Read the model definition and answer for the solid it produces. Units are mm, in the model's axes. Face numbers are marked on the shaded views. Round coordinates to 2 decimals unless told otherwise and drop trailing zeros. Loops run counter-clockwise (first coordinate to the right, second up) from the corner with the lowest first, then second, coordinate; pieces in that order, holes last. Notation, with made-up numbers: M -38,69 L 11,69 A11 ccw 11,87 Z; hole C 2.5,58.5 d4. An arc over 180 degrees is marked long. Write each question's results on one line, items separated by ' | '.
```python
from build123d import *

# Parameters (mm, degrees)
SKETCH1_R                  = 8.89
BOSS_EXTRUDE1_DEPTH        = 38.1
F_3_0MM_DOWEL_HOLE2_D      = 3.5
F_12_CLEARANCE_HOLE1_D     = 5.7912
F_12_CLEARANCE_HOLE1_DEPTH = 19.05
F_12_CLEARANCE_HOLE1_TIP   = 1.739852008


# Read off the part's stored shape, not the designer's step: CBORE for #2 Button Head Cap Screw1
with BuildPart() as part:
    # Sketch1 → Boss-Extrude1 (new body)
    with BuildSketch(Plane(origin=(0, 0, 0), x_dir=(1, 0, 0), z_dir=(0, 1, 0))):
        with Locations(Location((0, 0, 0), (0, 0, 90))):
            Circle(SKETCH1_R)
    extrude(amount=BOSS_EXTRUDE1_DEPTH)

    # Ø3.0mm Dowel Hole2 (through all)
    with Locations(Plane(origin=(0, 38.1, 0), x_dir=(1, 0, 0), z_dir=(0, 1, 0))):
        with Locations((0, 0)):
            Hole(F_3_0MM_DOWEL_HOLE2_D / 2)

    # CBORE for #2 Button Head Cap Screw1 outl → CBORE for #2 Button Head Cap Screw1 (revolve, cut)
    with BuildSketch(Plane(origin=(0, 5.08, 0), x_dir=(0, 1, 0), z_dir=(0, 0, -1))):
        Polygon((1.35255, 6.9596), (2.70637, 6.9596), (2.70637, 8.890055176), (0, 8.890055176), (0, 1.110061146), (1.35255, 1.110061146), align=None)
    revolve(axis=Axis((0, 5.08, 0), (1, 0, 0)), mode=Mode.SUBTRACT)

    # #12 Clearance Hole1
    with Locations(Plane(origin=(0, 38.1, 0), x_dir=(1, 0, 0), z_dir=(0, 1, 0))):
        with Locations((0, 0)):
            Hole(F_12_CLEARANCE_HOLE1_D / 2, depth=F_12_CLEARANCE_HOLE1_DEPTH)
            with Locations((0, 0, -(F_12_CLEARANCE_HOLE1_DEPTH + F_12_CLEARANCE_HOLE1_TIP / 2))):  # 118° drill point
                Cone(0, F_12_CLEARANCE_HOLE1_D / 2, F_12_CLEARANCE_HOLE1_TIP, mode=Mode.SUBTRACT)


solid = part.part
```
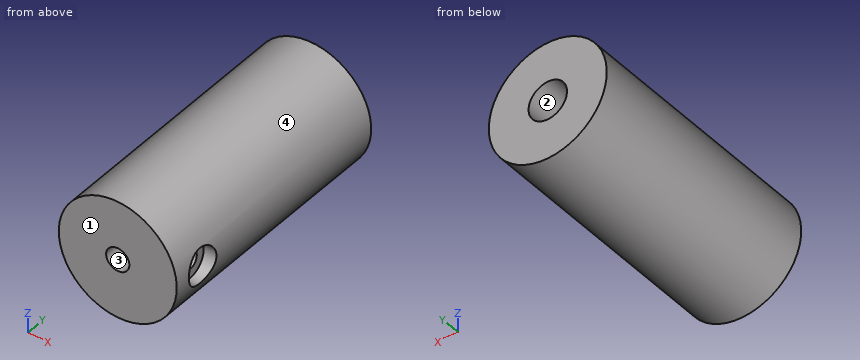
1. Given P1, Ø4, axis at y = 22.5, z = 5.5, coming from the +X side; P2, Ø2, axis at x = 2, y = 16.5, coming from the -Z side; P3, Ø2, axis at y = 18.5, z = -2, coming from the -X side, each flat-ended and moving along its own axis, determine where each tip first touches the part or whether it passes through.
Completed:
P1: stops at x = 8.17 | P2: stops at z = -8.83 | P3: stops at x = -8.83
2. Find the intervals of material crossed by L1, parallel to Y at x = 5.05, z = 0; L2, parallel to X at y = 25.5, z = 2.25; L3, parallel to Z at x = 5.2, y = 5.08, in increasing order.
Completed:
L1: y = 0 to 3.73, 6.43 to 38.1 | L2: x = -8.6 to -1.82, 1.82 to 8.6 | L3: z = -7.21 to -1.35, 1.35 to 7.21
3. Find section C-C, the plane y = 4.5. Give the vertices of the cut face in (x, z).
Completed:
outline: M 1.25,-1.22 A1.75 cw long 1.25,1.22 L 6.96,1.22 L 6.96,2.64 L 8.49,2.64 A8.89 ccw long 8.49,-2.64 L 6.96,-2.64 L 6.96,-1.22 Z
4. Find section D-D, the plane y = 17. Give the vertices of the cut face in (x, z).
Completed:
outline: C 0,0 d17.78; hole C 0,0 d3.5
5. Find section A-A, the plane z = 0. Give the vertices of the cut face in (x, y), then the cut area to 3 significant figures.
Completed:
outline: M -8.89,0 L -1.75,0 L -1.75,18.36 L -2.9,19.05 L -2.9,38.1 L -8.89,38.1 Z; M 1.75,0 L 8.89,0 L 8.89,2.37 L 6.96,2.37 L 6.96,3.73 L 1.75,3.73 Z; M 1.75,6.43 L 6.96,6.43 L 6.96,7.79 L 8.89,7.79 L 8.89,38.1 L 2.9,38.1 L 2.9,19.05 L 1.75,18.36 Z | area: 475 mm2
6. Find section B-B, the plane x = 0. Give the vertices of the cut face in (y, z).
Completed:
outline: M 0,-8.89 L 38.1,-8.89 L 38.1,-2.9 L 19.05,-2.9 L 18.36,-1.75 L 0,-1.75 Z; M 0,1.75 L 18.36,1.75 L 19.05,2.9 L 38.1,2.9 L 38.1,8.89 L 0,8.89 Z
7. Determine the mould class of the marked faces 1, 2, 3 and 4 for opening direction X: released by +X, released by -X, zero draft, split by the parting line, or undercut.
Completed:
face 1: zero draft | face 2: undercut | face 3: undercut | face 4: split by the parting line
